Verification items for the finished model (mm, model axes). Face numbers are marked on the shaded views. A direction names the side the tool comes from. Coordinates: 2 decimals unless noted, no trailing zeros. Write each loop counter-clockwise with the first axis right and the second up, starting at its lowest first coordinate (ties: lowest second). Pieces come first, ordered by that corner, then holes. Notation, with made-up numbers: (88, 79.25) -> (94, 79.25) arc R15 cw to (94, 96.25) -> close; hole circle Ø8 at (43, 36). An arc over 180 degrees is marked (long way). Answer in a Markdown table with one row per item.
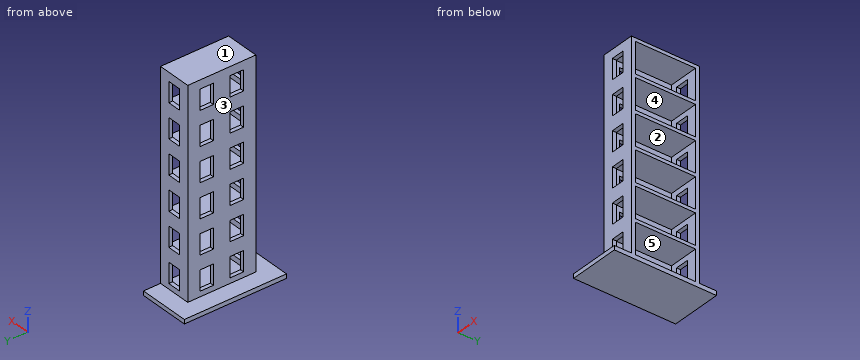
```python
from build123d import *

# Parameters (mm, degrees)
F0_W      = 30.48
F0_H      = 30.48
F1_DEPTH  = 1.27
F2_W      = 20.32
F2_H      = 20.32
F2_W_2    = 18
F2_H_2    = 18
F3_DEPTH  = 60.96
F5_DEPTH  = 74.4
F6_W      = 9
F6_H      = 1
F7_DEPTH  = 9
F8_W      = 4
F8_H      = 3
F9_DEPTH  = 53.6
F11_DEPTH = 68.5


with BuildPart() as f1:
    # F0 (on Top) → F1 (new body)
    with BuildSketch(Plane.XY):
        Rectangle(F0_W, F0_H)
    extrude(amount=F1_DEPTH)

    # F2 (on face) → F3 (join)
    with BuildSketch(Plane.XY.offset(1.27)):
        Rectangle(F2_W, F2_H)
        Rectangle(F2_W_2, F2_H_2, mode=Mode.SUBTRACT)
    extrude(amount=F3_DEPTH)

    # F4 (on Top) → F5 (cut)
    with BuildSketch(Plane.XY):
        Polygon((0, 23.4475191683), (0, -30.1982481033), (25.5301650614, -30.3230863065), (25.5301650614, 23.4475191683), align=None)
    extrude(amount=F5_DEPTH, mode=Mode.SUBTRACT)

    # F6 (on face) → F7 (join)
    with BuildSketch(Plane.YZ.offset(-9)):
        with Locations((-4.5, 10.93)):
            Rectangle(F6_W, F6_H)
        with Locations((-4.5, 61.73)):
            Rectangle(F6_W, F6_H)
        with Locations((4.5, 61.73)):
            Rectangle(F6_W, F6_H)
        with Locations((-4.5, 51.57)):
            Rectangle(F6_W, F6_H)
        with Locations((4.5, 51.57)):
            Rectangle(F6_W, F6_H)
        with Locations((-4.5, 41.41)):
            Rectangle(F6_W, F6_H)
        with Locations((4.5, 41.41)):
            Rectangle(F6_W, F6_H)
        with Locations((-4.5, 31.25)):
            Rectangle(F6_W, F6_H)
        with Locations((4.5, 31.25)):
            Rectangle(F6_W, F6_H)
        with Locations((-4.5, 21.09)):
            Rectangle(F6_W, F6_H)
        with Locations((4.5, 21.09)):
            Rectangle(F6_W, F6_H)
        with Locations((4.5, 10.93)):
            Rectangle(F6_W, F6_H)
    extrude(amount=F7_DEPTH)

    # F8 (on face) → F9 (cut)
    with BuildSketch(Plane.YZ):
        with Locations((4.5, 7.35)):
            Rectangle(F8_W, F8_H)
        with Locations((4.5, 4.35)):
            Rectangle(F8_W, F8_H)
        with Locations((-4.5, 4.35)):
            Rectangle(F8_W, F8_H)
        with Locations((-4.5, 7.35)):
            Rectangle(F8_W, F8_H)
        with Locations((-4.5, 14.51)):
            Rectangle(F8_W, F8_H)
        with Locations((-4.5, 17.51)):
            Rectangle(F8_W, F8_H)
        with Locations((-4.5, 24.67)):
            Rectangle(F8_W, F8_H)
        with Locations((-4.5, 27.67)):
            Rectangle(F8_W, F8_H)
        with Locations((4.5, 27.67)):
            Rectangle(F8_W, F8_H)
        with Locations((4.5, 24.67)):
            Rectangle(F8_W, F8_H)
        with Locations((4.5, 17.51)):
            Rectangle(F8_W, F8_H)
        with Locations((4.5, 14.51)):
            Rectangle(F8_W, F8_H)
        with Locations((4.5, 34.83)):
            Rectangle(F8_W, F8_H)
        with Locations((-4.5, 34.83)):
            Rectangle(F8_W, F8_H)
        with Locations((-4.5, 37.83)):
            Rectangle(F8_W, F8_H)
        with Locations((4.5, 37.83)):
            Rectangle(F8_W, F8_H)
        with Locations((-4.5, 55.15)):
            Rectangle(F8_W, F8_H)
        with Locations((-4.5, 58.15)):
            Rectangle(F8_W, F8_H)
        with Locations((4.5, 58.15)):
            Rectangle(F8_W, F8_H)
        with Locations((4.5, 55.15)):
            Rectangle(F8_W, F8_H)
        with Locations((4.5, 47.99)):
            Rectangle(F8_W, F8_H)
        with Locations((4.5, 44.99)):
            Rectangle(F8_W, F8_H)
        with Locations((-4.5, 44.99)):
            Rectangle(F8_W, F8_H)
        with Locations((-4.5, 47.99)):
            Rectangle(F8_W, F8_H)
    extrude(amount=-F9_DEPTH, mode=Mode.SUBTRACT)

    # F10 (on face) → F11 (cut)
    with BuildSketch(Plane.XZ.offset(10.16)):
        Polygon((-7.08, 34.5268503937), (-5.08, 36.33), (-7.08, 36.33), align=None)
        Polygon((-5.08, 33.33), (-5.08, 36.33), (-7.08, 34.5268503937), (-7.08, 33.33), align=None)
        Polygon((-3.08, 34.5268503937), (-5.08, 36.33), (-5.08, 33.33), (-3.08, 33.33), align=None)
        Polygon((-3.08, 34.5268503937), (-3.08, 36.33), (-5.08, 36.33), align=None)
        Polygon((-3.08, 36.33), (-3.08, 38.1331496063), (-5.08, 36.33), align=None)
        Polygon((-5.08, 36.33), (-3.08, 38.1331496063), (-3.08, 39.33), (-5.08, 39.33), align=None)
        Polygon((-7.08, 39.33), (-7.08, 38.1331496063), (-5.08, 36.33), (-5.08, 39.33), align=None)
        Polygon((-5.08, 36.33), (-7.08, 38.1331496063), (-7.08, 36.33), align=None)
        Polygon((-3.08, 44.6868503937), (-5.08, 46.49), (-5.08, 43.49), (-3.08, 43.49), align=None)
        Polygon((-3.08, 44.6868503937), (-3.08, 46.49), (-5.08, 46.49), align=None)
        Polygon((-3.08, 46.49), (-3.08, 48.2931496063), (-5.08, 46.49), align=None)
        Polygon((-5.08, 46.49), (-3.08, 48.2931496063), (-3.08, 49.49), (-5.08, 49.49), align=None)
        Polygon((-7.08, 49.49), (-7.08, 48.2931496063), (-5.08, 46.49), (-5.08, 49.49), align=None)
        Polygon((-5.08, 46.49), (-7.08, 48.2931496063), (-7.08, 46.49), align=None)
        Polygon((-7.08, 44.6868503937), (-5.08, 46.49), (-7.08, 46.49), align=None)
        Polygon((-5.08, 43.49), (-5.08, 46.49), (-7.08, 44.6868503937), (-7.08, 43.49), align=None)
        Polygon((-5.08, 53.65), (-5.08, 56.65), (-7.08, 54.8468503937), (-7.08, 53.65), align=None)
        Polygon((-7.08, 54.8468503937), (-5.08, 56.65), (-7.08, 56.65), align=None)
        Polygon((-7.08, 56.65), (-5.08, 56.65), (-7.08, 58.4531496063), align=None)
        Polygon((-5.08, 56.65), (-5.08, 59.65), (-7.08, 59.65), (-7.08, 58.4531496063), align=None)
        Polygon((-3.08, 59.65), (-5.08, 59.65), (-5.08, 56.65), (-3.08, 58.4531496063), align=None)
        Polygon((-3.08, 58.4531496063), (-5.08, 56.65), (-3.08, 56.65), align=None)
        Polygon((-3.08, 56.65), (-5.08, 56.65), (-3.08, 54.8468503937), align=None)
        Polygon((-3.08, 54.8468503937), (-5.08, 56.65), (-5.08, 53.65), (-3.08, 53.65), align=None)
        Polygon((-3.08, 24.3668503937), (-5.08, 26.17), (-5.08, 23.17), (-3.08, 23.17), align=None)
        Polygon((-5.08, 23.17), (-5.08, 26.17), (-7.08, 24.3668503937), (-7.08, 23.17), align=None)
        Polygon((-7.08, 29.17), (-7.08, 27.9731496063), (-5.08, 26.17), (-5.08, 29.17), align=None)
        Polygon((-5.08, 26.17), (-3.08, 27.9731496063), (-3.08, 29.17), (-5.08, 29.17), align=None)
        Polygon((-3.08, 24.3668503937), (-3.08, 26.17), (-5.08, 26.17), align=None)
        Polygon((-3.08, 26.17), (-3.08, 27.9731496063), (-5.08, 26.17), align=None)
        Polygon((-5.08, 26.17), (-7.08, 27.9731496063), (-7.08, 26.17), align=None)
        Polygon((-7.08, 24.3668503937), (-5.08, 26.17), (-7.08, 26.17), align=None)
        Polygon((-7.08, 19.01), (-7.08, 17.8131496063), (-5.08, 16.01), (-5.08, 19.01), align=None)
        Polygon((-5.08, 16.01), (-7.08, 17.8131496063), (-7.08, 16.01), align=None)
        Polygon((-7.08, 14.2068503937), (-5.08, 16.01), (-7.08, 16.01), align=None)
        Polygon((-5.08, 13.01), (-5.08, 16.01), (-7.08, 14.2068503937), (-7.08, 13.01), align=None)
        Polygon((-3.08, 14.2068503937), (-5.08, 16.01), (-5.08, 13.01), (-3.08, 13.01), align=None)
        Polygon((-3.08, 14.2068503937), (-3.08, 16.01), (-5.08, 16.01), align=None)
        Polygon((-3.08, 16.01), (-3.08, 17.8131496063), (-5.08, 16.01), align=None)
        Polygon((-5.08, 16.01), (-3.08, 17.8131496063), (-3.08, 19.01), (-5.08, 19.01), align=None)
        Polygon((-7.08, 8.85), (-7.08, 7.6531496063), (-5.08, 5.85), (-5.08, 8.85), align=None)
        Polygon((-5.08, 5.85), (-3.08, 7.6531496063), (-3.08, 8.85), (-5.08, 8.85), align=None)
        Polygon((-3.08, 5.85), (-3.08, 7.6531496063), (-5.08, 5.85), align=None)
        Polygon((-3.08, 4.0468503937), (-3.08, 5.85), (-5.08, 5.85), align=None)
        Polygon((-3.08, 4.0468503937), (-5.08, 5.85), (-5.08, 2.85), (-3.08, 2.85), align=None)
        Polygon((-5.08, 2.85), (-5.08, 5.85), (-7.08, 4.0468503937), (-7.08, 2.85), align=None)
        Polygon((-7.08, 4.0468503937), (-5.08, 5.85), (-7.08, 5.85), align=None)
        Polygon((-5.08, 5.85), (-7.08, 7.6531496063), (-7.08, 5.85), align=None)
    extrude(amount=-F11_DEPTH, mode=Mode.SUBTRACT)


solid = f1.part
```
1. Access from +Z, -Z, +X, -X, +Y, -Y to the whole of each face (thin tool, end or side, straight path). Record for the marked faces 1 and 2.
Findings below:
| item | result |
|---|---|
| face 1 | +Z, +X, -X, +Y, -Y |
| face 2 | +X |
2. Go/stop test with flat-tipped pins: pin 1 (6 mm diameter, centred on x = -4, z = 26.5, fed in from -Y); pin 2 (0.9 mm diameter, centred on x = -9.5, z = 36.5, fed in from +Y); pin 3 (1.3 mm diameter, centred on y = -9.5, z = 56, fed in from -X). Record where each tip stops, or that it passes through.
Findings below:
| item | result |
|---|---|
| pin 1 | stops at y = -10.16 |
| pin 2 | stops at y = 10.16 |
| pin 3 | stops at x = -10.16 |
3. Sectioned sample at B-B, the plane x = -1.25. Count the separate pieces of the cut face and the enclosed holes in it, and give its area (3 significant figures).
Findings below:
| item | result |
|---|---|
| separate pieces | 1 |
| enclosed holes | 6 |
| area | 288 mm² |
4. Release check for a two-part mould opening along Y. For the marked faces 3, 4 and 5 record: released by +Y, released by -Y, zero draft, split by the parting line, or undercut.
Findings below:
| item | result |
|---|---|
| face 3 | zero draft |
| face 4 | undercut |
| face 5 | undercut |
5. Material ranges on probe 1 along Y at (x, z) = (-9.25, 59.5); probe 2 along Y at (x, z) = (-4.5, 50.5); probe 3 along X at (y, z) = (7.5, 5.5), recorded low to high. Write a range as from..to.
Findings below:
| item | result |
|---|---|
| probe 1 | y = -10.16..-6.5, -2.5..2.5, 6.5..10.16 |
| probe 2 | y = -10.16..-9, 9..10.16 |
| probe 3 | x = -10.16..-9 |
6. Sectioned sample at A-A, the plane z = 5. Record the cut outline in (x, y), and give its area (3 significant figures).
Findings below:
| item | result |
|---|---|
| outline | (-10.16, -10.16) -> (-7.08, -10.16) -> (-7.08, -9) -> (-9, -9) -> (-9, -6.5) -> (-10.16, -6.5) -> close; (-10.16, -2.5) -> (-9, -2.5) -> (-9, 2.5) -> (-10.16, 2.5) -> close; (-10.16, 6.5) -> (-9, 6.5) -> (-9, 9) -> (-7.08, 9) -> (-7.08, 10.16) -> (-10.16, 10.16) -> close; (-3.08, -10.16) -> (0, -10.16) -> (0, -9) -> (-3.08, -9) -> close; (-3.08, 9) -> (0, 9) -> (0, 10.16) -> (-3.08, 10.16) -> close |
| area | 25.9 mm² |
